```python
from build123d import *

# Parameters (mm, degrees)
F0_W     = 68.58
F0_H     = 25.4
F1_DEPTH = 25.4
F2_W     = 25.4
F2_H     = 25.4
F3_DEPTH = 17.78
F4_W     = 25.4
F4_H     = 17.78
F5_DEPTH = 50.8
F6_W     = 25.4
F6_H     = 25.4
F7_DEPTH = 25.4


with BuildPart() as f1:
    # F0 (on Right) → F1 (new body)
    with BuildSketch(Plane.YZ):
        with Locations((43.169466, 18.918027)):
            Rectangle(F0_W, F0_H)
    extrude(amount=F1_DEPTH)

    # F2 (on face) → F3 (join)
    with BuildSketch(Plane.XY.offset(31.618027)):
        with Locations((12.7, 21.579466)):
            Rectangle(F2_W, F2_H)
    extrude(amount=F3_DEPTH)

    # F4 (on face) → F5 (join)
    with BuildSketch(Plane.YZ.offset(25.4)):
        with Locations((21.579466, 40.508027)):
            Rectangle(F4_W, F4_H)
    extrude(amount=F5_DEPTH)

    # F6 (on face) → F7 (join)
    with BuildSketch(Plane(origin=(0, 0, 31.618027), x_dir=(1, 0, 0), z_dir=(0, 0, -1))):
        with Locations((63.5, -21.579466)):
            Rectangle(F6_W, F6_H)
    extrude(amount=F7_DEPTH)


solid = f1.part
```
Read the model definition and answer for the solid it produces. Units are mm, in the model's axes. A direction names the side the tool comes from. Give positions to 0.01 mm unless a question says otherwise; leave off trailing zeros. Order: outer loops, then holes, each group sorted by start corner. A loop starts at its lowest first (then second) coordinate and runs counter-clockwise, first axis right, second up. Notation, with made-up numbers: (1, 14) -> (58, 14) arc R9 ccw to (58, 28) -> close; hole circle Ø5 at (49.5, 7.5). An arc over 180 degrees is marked (long way). One line per item, written item: value. Start each with the question number.
(1) The part is cut by section D-D (y = 60). Determine the outline of the cut face in (x, z).
(2) Straight lines are drawn through the part: L1, parallel to X at y = 17, z = 24.5; L2, parallel to Y at x = 20.5, z = 40.5; L3, parallel to Z at x = 17, y = 71.5. For each, find the intervals that lie inside material, in ascending order.
(3) A tool of negligible diameter and unlimited length cuts with its end or side. For faces 5 (the flat face through (46, 34.279, 33)), 6 (the flat face through (13, 56, 31.618)), 7 (the flat face through (25.4, 43, 19)), from which of +Z, -Z, +X, -X, +Y, -Y can it reach the whole face along a straight path? Write none if from no direction.
(4) The part is cut by section B-B (y = 21.5). Determine the outline of the cut face in (x, z), and give its area (3 significant figures).
(5) The part is cut by section C-C (x = 16.5). Determine the outline of the cut face in (y, z), and give its area (3 significant figures).
(6) Flat-ended cylindrical pins translate along their axes: P1, Ø12, axis at x = 30, z = 14, coming from the -Y side; P2, Ø3, axis at y = 56, z = 32, coming from the +X side; P3, Ø1.5, axis at x = 35, z = 32, coming from the +Y side; P4, Ø20.5, axis at x = 7, y = 59.5, coming from the +Z side. Find the tip coordinate at first contact, or state that the pin passes through.
(7) For a pull along X with two mould halves and no side action, classify faces 1 (the flat face through (50.8, 22, 19)), 2 (the flat face through (38, 21, 31.618)), 3 (the flat face through (76.2, 22, 28)), 4 (the flat face through (38, 8.879, 33)) as released by +X, released by -X, zero draft, split by the parting line, or undercut.
(8) The part is cut by section A-A (z = 17). Determine the outline of the cut face in (x, y).
Taken from the geometry:
1. outline: (0, 6.22) -> (25.4, 6.22) -> (25.4, 31.62) -> (0, 31.62) -> close
2. L1: 0 to 25.4, 50.8 to 76.2
2. L2: 8.88 to 34.28
2. L3: 6.22 to 31.62
3. face 5: +Z, +X, +Y
3. face 6: +Z, +X, -X, +Y
3. face 7: -Z, +Y, -Y
4. outline: (0, 6.22) -> (25.4, 6.22) -> (25.4, 31.62) -> (50.8, 31.62) -> (50.8, 6.22) -> (76.2, 6.22) -> (76.2, 49.4) -> (0, 49.4) -> close
4. area: 2,650 mm^2
5. outline: (8.88, 6.22) -> (77.46, 6.22) -> (77.46, 31.62) -> (34.28, 31.62) -> (34.28, 49.4) -> (8.88, 49.4) -> close
5. area: 2,190 mm^2
6. P1: y = 8.88
6. P2: x = 25.4
6. P3: y = 34.28
6. P4: z = 31.62
7. face 1: undercut
7. face 2: undercut
7. face 3: released by +X
7. face 4: zero draft
8. outline: (0, 8.88) -> (25.4, 8.88) -> (25.4, 77.46) -> (0, 77.46) -> close; (50.8, 8.88) -> (76.2, 8.88) -> (76.2, 34.28) -> (50.8, 34.28) -> close
